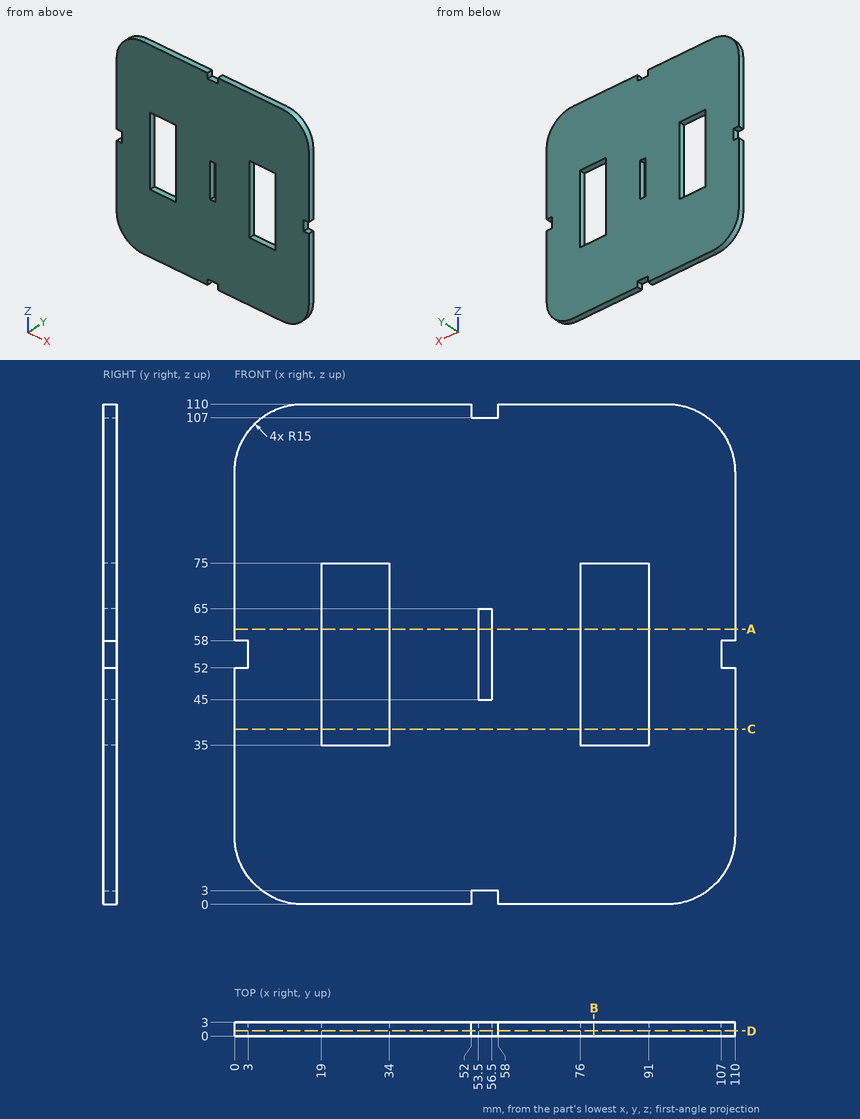
Study the drawing (mm; zero at the part's minimum x, y, z) and answer. Give positions to 0.01 mm unless a question says otherwise; leave off trailing zeros. Write each loop counter-clockwise with the first axis right and the second up, starting at its lowest first coordinate (ties: lowest second). Pieces come first, ordered by that corner, then holes. Notation, with made-up numbers: (36, 20.25) - (91, 20.25) arc R24 cw to (91, 40.25) - close; hole circle Ø10 at (-21.5, 1.25). An arc over 180 degrees is marked (long way). Write item = value, one per line. Start each with the question number.
Item 1: Find the intervals of material crossed by probe 1 along X at (y, z) = (2.75, 41); probe 2 along X at (y, z) = (2.1, 46.5); probe 3 along Z at (x, y) = (22, 1.7), in increasing order. Write a range as [from, to].
Item 2: Find section A-A (z = 60.5). Give the vertices of the cut face in (x, y), then the cut area to 3 significant figures.
Item 3: Find section B-B (x = 79). Give the vertices of the cut face in (y, z).
Item 4: Each of these flat-tipped pins is pushed along its axis until it touches: P1, Ø1.5, axis at y = 2, z = 54.5, coming from the +X side; P2, Ø1.5, axis at x = 28, y = 1, coming from the -Z side; P3, Ø1.5, axis at x = 108, y = 1.5, coming from the -Z side; P4, Ø0.9, axis at x = 1, y = 2, coming from the +Z side. Where does it stop, or does it pass through?
Item 5: Find section C-C (z = 38.5). Give the vertices of the cut face in (x, y).
Item 6: Find section D-D (y = 1.1). State how many separate pieces and enclosed holes the cut face has, then the cut area to 3 significant figures.
Response:
q1.probe_1 = [0, 19], [34, 76], [91, 110]
q1.probe_2 = [0, 19], [34, 53.5], [56.5, 76], [91, 110]
q1.probe_3 = [0, 35], [75, 110]
q2.outline = (0, 0) - (19, 0) - (19, 3) - (0, 3) - close; (34, 0) - (53.5, 0) - (53.5, 3) - (34, 3) - close; (56.5, 0) - (76, 0) - (76, 3) - (56.5, 3) - close; (91, 0) - (110, 0) - (110, 3) - (91, 3) - close
q2.area = 231 mm²
q3.outline = (0, 0) - (3, 0) - (3, 35) - (0, 35) - close; (0, 75) - (3, 75) - (3, 110) - (0, 110) - close
q4.P1 = 107
q4.P2 = 0
q4.P3 = 6.34
q4.P4 = 101.43
q5.outline = (0, 0) - (19, 0) - (19, 3) - (0, 3) - close; (34, 0) - (76, 0) - (76, 3) - (34, 3) - close; (91, 0) - (110, 0) - (110, 3) - (91, 3) - close
q6.separate_pieces = 1
q6.enclosed_holes = 3
q6.area = 10,600 mm²
